The listing builds one solid part. Answer for the finished solid, in the listing's coordinates (mm). Face numbers are marked on the shaded views. A direction names the side the tool comes from. Round coordinates to 2 decimals unless told otherwise and drop trailing zeros. Write each loop counter-clockwise with the first axis right and the second up, starting at its lowest first coordinate (ties: lowest second). Pieces come first, ordered by that corner, then holes. Notation, with made-up numbers: (34, -31) - (42, -31) arc R22 cw to (42, 4) - close; hole circle Ø4 at (-35, 37). An arc over 180 degrees is marked (long way). Answer in a Markdown table with one row per item.
from build123d import *

# Parameters (mm, degrees)
SKETCH1_W           = 5
SKETCH1_H           = 5
BOSS_EXTRUDE2_DEPTH = 45


with BuildPart() as part:
    # Sketch1 → Boss-Extrude2 (new body)
    with BuildSketch(Plane(origin=(0, 0, 0), x_dir=(0, 0, -1), z_dir=(1, 0, 0))):
        Polygon((-10, 10), (-3, 10), (-3, 8.5), (-6, 8.5), (-6, 7.5), (-3, 4.5), (-0.75, 4.5), (0, 3.75), (0.75, 4.5), (3, 4.5), (6, 7.5), (6, 8.5), (3, 8.5), (3, 10), (10, 10), (10, 3), (8.5, 3), (8.5, 6), (7.5, 6), (4.5, 3), (4.5, 0.75), (3.75, 0), (4.5, -0.75), (4.5, -3), (7.5, -6), (8.5, -6), (8.5, -3), (10, -3), (10, -10), (3, -10), (3, -8.5), (6, -8.5), (6, -7.5), (3, -4.5), (0.75, -4.5), (0, -3.75), (-0.75, -4.5), (-3, -4.5), (-6, -7.5), (-6, -8.5), (-3, -8.5), (-3, -10), (-10, -10), (-10, -3), (-8.5, -3), (-8.5, -6), (-7.5, -6), (-4.5, -3), (-4.5, -0.75), (-3.75, 0), (-4.5, 0.75), (-4.5, 3), (-7.5, 6), (-8.5, 6), (-8.5, 3), (-10, 3), align=None)
        Rectangle(SKETCH1_W, SKETCH1_H, mode=Mode.SUBTRACT)
    extrude(amount=BOSS_EXTRUDE2_DEPTH)


solid = part.part
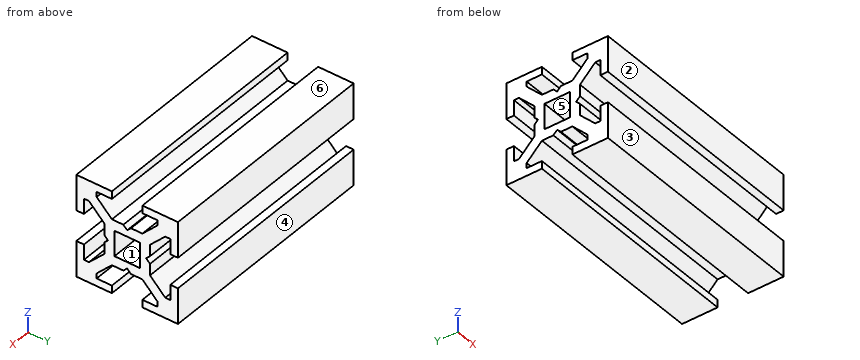
(1) Section C-C (z = 5) is taken. Give the vertices of the cut face in (x, y), and give its area (3 significant figures).
Checked values:
| item | result |
|---|---|
| outline | (0, -10) - (45, -10) - (45, -8.5) - (0, -8.5) - close; (0, -6.5) - (45, -6.5) - (45, -3.5) - (0, -3.5) - close; (0, 3.5) - (45, 3.5) - (45, 6.5) - (0, 6.5) - close; (0, 8.5) - (45, 8.5) - (45, 10) - (0, 10) - close |
| area | 405 mm2 |
(2) For the marked faces 1 and 2, determine the directions among +Z, -Z, +X, -X, +Y, -Y from which every point of the face is accessible in a straight line to the end or side of a thin tool.
Checked values:
| item | result |
|---|---|
| face 1 | +X, -X |
| face 2 | +Z, -Z, +X, -X, -Y |
(3) Find the intervals of material crossed by line 1 (Y direction, x = 35, z = -2.25); line 2 (Y direction, x = 38.5, z = -9); line 3 (Y direction, x = 18, z = -5.5), in increasing order.
Checked values:
| item | result |
|---|---|
| line 1 | y = -4.5 to -2.5, 2.5 to 4.5 |
| line 2 | y = -10 to -3, 3 to 10 |
| line 3 | y = -10 to -8.5, -7 to -4, 4 to 7, 8.5 to 10 |
(4) For a pull along Y with two mould halves and no side action, classify the marked faces 3, 4, 5 and 6 as pulls with the +Y half, pulls with the -Y half, needs draft (parallel to the pull), parting line crosses it, or undercut.
Checked values:
| item | result |
|---|---|
| face 3 | pulls with the -Y half |
| face 4 | pulls with the +Y half |
| face 5 | undercut |
| face 6 | needs draft |
(5) A flat-ended cylindrical pin translates along its axis: pin 1 (1.5 mm diameter, centred on x = 21, y = -0.5, fed in from -Z). Find the tip coordinate at first contact, or state that the pin passes through.
Checked values:
| item | result |
|---|---|
| pin 1 | stops at z = -4.5 |
(6) Section A-A (y = 1.75) is taken. Give the vertices of the cut face in (x, z).
Checked values:
| item | result |
|---|---|
| outline | (0, -4.5) - (45, -4.5) - (45, -2.5) - (0, -2.5) - close; (0, 2.5) - (45, 2.5) - (45, 4.5) - (0, 4.5) - close |
